```python
from build123d import *

# Parameters (mm, degrees)
BOSS_EXTRUDE2_DEPTH                               = 4.7625
F_4_CLEARANCE_HOLE1_D                             = 3.2639
CSK_FOR_4_FLAT_HEAD_SOCKET_CAP_SCREW2_D           = 3.2639
CSK_FOR_4_FLAT_HEAD_SOCKET_CAP_SCREW2_CSINK_D     = 6.477
CSK_FOR_4_FLAT_HEAD_SOCKET_CAP_SCREW2_CSINK_ANGLE = 82


with BuildPart() as part:
    # Sketch1 → Boss-Extrude2 (new body)
    with BuildSketch(Plane(origin=(0, 0, 0), x_dir=(1, 0, 0), z_dir=(0, 1, 0))):
        with BuildLine():
            Line((-63.5, 6.35), (0, 6.35))
            ThreePointArc((0, 6.35), (6.35, 0), (0, -6.35))
            Line((0, -6.35), (-63.5, -6.35))
            ThreePointArc((-63.5, -6.35), (-69.85, 0), (-63.5, 6.35))
        make_face()
    extrude(amount=BOSS_EXTRUDE2_DEPTH)

    # #4 Clearance Hole1 (through all)
    with Locations(Plane(origin=(0, 4.7625, 0), x_dir=(1, 0, 0), z_dir=(0, 1, 0))):
        with Locations((-63.5, 0)):
            Hole(F_4_CLEARANCE_HOLE1_D / 2)

    # CSK for #4 Flat Head Socket Cap Screw2 (through all)
    with Locations(Plane(origin=(0, 0, 0), x_dir=(-1, 0, 0), z_dir=(0, -1, 0))):
        with Locations((0, 0)):
            CounterSinkHole(CSK_FOR_4_FLAT_HEAD_SOCKET_CAP_SCREW2_D / 2, CSK_FOR_4_FLAT_HEAD_SOCKET_CAP_SCREW2_CSINK_D / 2, counter_sink_angle=CSK_FOR_4_FLAT_HEAD_SOCKET_CAP_SCREW2_CSINK_ANGLE)


solid = part.part
```
For this review, take the finished solid that the model builds, in its own axes (mm). Coordinates: 2 decimals unless noted, no trailing zeros. Write each loop counter-clockwise with the first axis right and the second up, starting at its lowest first coordinate (ties: lowest second). Pieces come first, ordered by that corner, then holes. Notation, with made-up numbers: (-2, 22.5) - (53, 22.5) arc R17 cw to (53, 46.5) - close; hole circle Ø1 at (49, -22.5). An arc over 180 degrees is marked (long way). Answer in a Markdown table with one row per item. Add a question column.
Q1. We need section C-C, the plane z = 4. State the section outline as (x, y) points.
Q2. We need section A-A, the plane z = 0. State the section outline as (x, y) points.
Q3. We need section B-B, the plane y = 4. State the section outline as (x, z) points.
Q4. For P1, Ø1.5, axis at y = 2.5, z = -4.5, coming from the -X side, flat-tipped, find the tip position at first contact; note if it passes through.
Q5. For probe 1 along Z at (x, y) = (-63.5, 1.95); probe 2 along X at (y, z) = (2.2, -1.25); probe 3 along X at (y, z) = (1.3, 1), list the stretches that pass through material, from the lowest coordinate up.
Q6. Draft analysis for pull direction X (two halves, no side actions). For faces 1 (the cylindrical face through (6.35, 2.35, -0.14)), 2 (the cylindrical face through (-0.354, 3.326, 1.593)), 3 (the flat face through (-32, 2, -6.35)), state which applies: +X half, -X half, draft (parallel to the pull), parting line (faces both ways), or undercut.
Answer list:
| question | item | result |
|---|---|---|
| 1 | outline | (-68.43, 0) - (4.93, 0) - (4.93, 4.76) - (-68.43, 4.76) - close |
| 2 | outline | (-69.85, 0) - (-65.13, 0) - (-65.13, 4.76) - (-69.85, 4.76) - close; (-61.87, 0) - (-3.24, 0) - (-1.63, 1.85) - (-1.63, 4.76) - (-61.87, 4.76) - close; (1.63, 1.85) - (3.24, 0) - (6.35, 0) - (6.35, 4.76) - (1.63, 4.76) - close |
| 3 | outline | (-63.5, -6.35) - (0, -6.35) arc R6.35 ccw to (0, 6.35) - (-63.5, 6.35) arc R6.35 ccw to start; hole circle Ø3.26 at (-63.5, 0); hole circle Ø3.26 at (0, 0) |
| 4 | P1 | stops at x = -68.62 |
| 5 | probe 1 | z = -6.35 to -1.63, 1.63 to 6.35 |
| 5 | probe 2 | x = -69.73 to -64.55, -62.45 to -1.05, 1.05 to 6.23 |
| 5 | probe 3 | x = -69.77 to -64.79, -62.21 to -1.86, 1.86 to 6.27 |
| 6 | face 1 | +X half |
| 6 | face 2 | undercut |
| 6 | face 3 | draft |
